Can you work these out from the model? Positions are in its coordinate system, mm. Give positions to 0.01 mm unless a question says otherwise; leave off trailing zeros. Loops run counter-clockwise (first coordinate to the right, second up) from the corner with the lowest first, then second, coordinate; pieces in that order, holes last. Notation, with made-up numbers: (83.5, 35) - (137.5, 35) arc R31 cw to (137.5, 60) - close; hole circle Ø7 at (55, -5). An arc over 180 degrees is marked (long way). Use a Markdown table: item, result. Add a question column.
```python
from build123d import *

# Parameters (mm, degrees)
BOSS_EXTRUDE1_DEPTH = 2.54
SKETCH2_R           = 1.651
CUT_EXTRUDE1_DEPTH  = 3.54
CIRPATTERN1_COUNT   = 6


with BuildPart() as part:
    # Sketch1 → Boss-Extrude1 (new body)
    with BuildSketch(Plane(origin=(0, 0, 0), x_dir=(1, 0, 0), z_dir=(0, 1, 0))):
        Polygon((43.884105286, -76.0095), (87.768210572, 0), (43.884105286, 76.0095), (-43.884105286, 76.0095), (-87.768210572, 0), (-43.884105286, -76.0095), align=None)
    extrude(amount=BOSS_EXTRUDE1_DEPTH)

    # Sketch2 → Cut-Extrude1 (cut, through all)
    with BuildSketch(Plane(origin=(0, 2.54, 0), x_dir=(1, 0, 0), z_dir=(0, 1, 0))):
        with Locations((-40.264605286, 69.740342102)):
            Circle(SKETCH2_R)
    cut_extrude1 = extrude(amount=-CUT_EXTRUDE1_DEPTH, mode=Mode.SUBTRACT)

    # CirPattern1: Cut-Extrude1 ×6 about axis
    cirpattern1_axis = Axis((0.017235622, 0, 0.029852973), (0, 1, 0))
    for i in range(1, CIRPATTERN1_COUNT):
        add(cut_extrude1.rotate(cirpattern1_axis, i * 360 / CIRPATTERN1_COUNT), mode=Mode.SUBTRACT)


solid = part.part
```
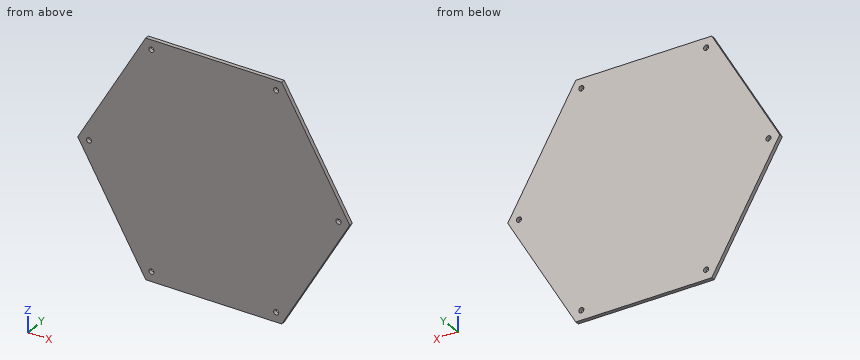
1. Please list where these lines run through material, in increasing order: line 1 along X through (y, z) = (0.75, 68.5); line 2 along X through (y, z) = (2, -1); line 3 along X through (y, z) = (0.8, 11). Write a range as [from, to].
2. Suppose I cut it at B-B (z = -51). List the corners of the cut face in (x, y) for me.
3. Will this pin go through, and if not, where does the flat tip stop? P1, Ø2, axis at x = -40.26, z = -69.74, coming from the +Y side.
4. Suppose I cut it at A-A (y = 0.4). List the corners of the cut face in (x, z) for me, and give its area (3 significant figures).
5. Suppose I cut it at C-C (x = 67.5). List the corners of the cut face in (y, z) for me.
Results below:
| question | item | result |
|---|---|---|
| 1 | line 1 | [-48.22, -41.28], [-39.25, 39.28], [41.32, 48.22] |
| 1 | line 2 | [-87.19, -81.84], [-79.26, 79.29], [81.87, 87.19] |
| 1 | line 3 | [-81.42, 81.42] |
| 2 | outline | (-58.32, 0) - (58.32, 0) - (58.32, 2.54) - (-58.32, 2.54) - close |
| 3 | P1 | through |
| 4 | outline | (-87.77, 0) - (-43.88, -76.01) - (43.88, -76.01) - (87.77, 0) - (43.88, 76.01) - (-43.88, 76.01) - close; hole circle Ø3.3 at (-80.55, 0.03); hole circle Ø3.3 at (-40.26, -69.74); hole circle Ø3.3 at (-40.26, 69.8); hole circle Ø3.3 at (40.3, -69.74); hole circle Ø3.3 at (40.3, 69.8); hole circle Ø3.3 at (80.58, 0.03) |
| 4 | area | 20,000 mm² |
| 5 | outline | (0, -35.11) - (2.54, -35.11) - (2.54, 35.11) - (0, 35.11) - close |
